Can you work these out from the model? Positions are in its coordinate system, mm. A direction names the side the tool comes from. Give positions to 0.01 mm unless a question says otherwise; leave off trailing zeros. Order: outer loops, then holes, each group sorted by start corner. A loop starts at its lowest first (then second) coordinate and runs counter-clockwise, first axis right, second up. Notation, with made-up numbers: M 64.25,80 L 117.25,80 A30 ccw 117.25,117 Z; hole C 33,24.5 d11. An arc over 180 degrees is marked long. Write each question's results on one line, items separated by ' | '.
from build123d import *

# Parameters (mm, degrees)
CROQUIS1_W              = 30
CROQUIS1_H              = 30
SALIENTE_EXTRUIR1_DEPTH = 3
CROQUIS2_R              = 1.5
CORTAR_EXTRUIR1_DEPTH   = 3


with BuildPart() as part:
    # Croquis1 → Saliente-Extruir1 (new body)
    with BuildSketch(Plane.XY):
        Rectangle(CROQUIS1_W, CROQUIS1_H)
        with BuildLine():
            Line((-6.418498959, -11), (1, -11))
            ThreePointArc((1, -11), (8.071067812, -8.071067812), (11, -1))
            Line((11, -1), (11, 6.418498959))
            ThreePointArc((11, 6.418498959), (10.640885104, 6.898239917), (10.07939445, 6.688852377))
            ThreePointArc((10.07939445, 6.688852377), (2.596324807, -2.596324807), (-6.688852377, -10.07939445))
            ThreePointArc((-6.688852377, -10.07939445), (-6.898239917, -10.640885104), (-6.418498959, -11))
        make_face(mode=Mode.SUBTRACT)
        with BuildLine():
            Line((-11, -6.418498959), (-11, 1))
            ThreePointArc((-11, 1), (-8.071067812, 8.071067812), (-1, 11))
            Line((-1, 11), (6.418498959, 11))
            ThreePointArc((6.418498959, 11), (6.898239917, 10.640885104), (6.688852377, 10.07939445))
            ThreePointArc((6.688852377, 10.07939445), (-2.596324807, 2.596324807), (-10.07939445, -6.688852377))
            ThreePointArc((-10.07939445, -6.688852377), (-10.640885104, -6.898239917), (-11, -6.418498959))
        make_face(mode=Mode.SUBTRACT)
    extrude(amount=SALIENTE_EXTRUIR1_DEPTH)

    # Croquis2 → Cortar-Extruir1 (cut)
    with BuildSketch(Plane.XY.offset(3)):
        with Locations((-10.378302419, -10.798607502)):
            Circle(CROQUIS2_R)
    extrude(amount=-CORTAR_EXTRUIR1_DEPTH, mode=Mode.SUBTRACT)


solid = part.part
(1) I need wall thicknesses on L1, parallel to Y at x = 1.25, z = 0.35; L2, parallel to Y at x = -2.5, z = 0.95; L3, parallel to X at y = 1, z = 2.3. Which ranges of each line are inside material? Lowest first, please. Write a range as from..to.
Data:
L1: y = -15..-11, -3.9..6.1, 11..15 | L2: y = -15..-11, -7.11..2.69, 10.89..15 | L3: x = -15..-11, -4.13..5.89, 11..15
(2) Imagine slicing it at C-C, the plane y = 0. Write out the boundary of the cut face in (x, z), plus the area to 3 significant figures.
Data:
outline: M -15,0 L -11,0 L -11,3 L -15,3 Z; M -5.03,0 L 5.03,0 L 5.03,3 L -5.03,3 Z; M 11,0 L 15,0 L 15,3 L 11,3 Z | area: 54.2 mm2
(3) Imagine slicing it at D-D, the plane z = 1. Write out the boundary of the cut face in (x, y), plus the area to 3 significant figures.
Data:
outline: M -15,-15 L 15,-15 L 15,15 L -15,15 Z; hole C -10.38,-10.8 d3; hole M -11,-6.42 A0.5 ccw -10.08,-6.69 A55.8 cw 6.69,10.08 A0.5 ccw 6.42,11 L -1,11 A10 ccw -11,1 Z; hole M -6.69,-10.08 A0.5 ccw -6.42,-11 L 1,-11 A10 ccw 11,-1 L 11,6.42 A0.5 ccw 10.08,6.69 A55.8 cw Z | area: 631 mm2
(4) We'd pull the mould along Y, two halves only. Please class faces 3 (the face through (-11, -3, 1)), 4 (the face through (0, 15, 1)), 5 (the face through (-15, 0, 1)), 6 (the face through (-2.48, 2.71, 1.48)): +Y half, -Y half, draft (parallel to the pull), parting line (faces both ways), or undercut.
Data:
face 3: undercut | face 4: +Y half | face 5: draft | face 6: undercut
(5) For faces 1 (the face through (0, 0, 0)), 2 (the face through (3, 11, 1)), which set-ups out of +Z, -Z, +X, -X, +Y, -Y let a thin tool reach every point of the face, with its end or its side?
Data:
face 1: -Z, +X, -X, +Y, -Y | face 2: +Z, -Z
(6) Imagine slicing it at B-B, the plane x = -4.25. Write out the boundary of the cut face in (y, z).
Data:
outline: M -15,0 L -11,0 L -11,3 L -15,3 Z; M -8.42,0 L 0.87,0 L 0.87,3 L -8.42,3 Z; M 10.46,0 L 15,0 L 15,3 L 10.46,3 Z
(7) Imagine slicing it at A-A, the plane y = 7.75. Write out the boundary of the cut face in (x, z).
Data:
outline: M -15,0 L -8.38,0 L -8.38,3 L -15,3 Z; M 3.34,0 L 15,0 L 15,3 L 3.34,3 Z
